from build123d import *

# Parameters (mm, degrees)
SKETCH2_W           = 219.964
SKETCH2_H           = 149.86
SKETCH1_W           = 190.5
SKETCH1_H           = 116.84
SKETCH2_2_W         = 219.964
SKETCH2_2_H         = 149.86
BOSS_EXTRUDE2_DEPTH = 4.572
SKETCH3_W           = 177.8
SKETCH3_H           = 109.22
BOSS_EXTRUDE3_DEPTH = 5.08
SKETCH4_W           = 167.64
SKETCH4_H           = 99.06
CUT_EXTRUDE1_DEPTH  = 6.08
SKETCH4_2_W         = 167.64
SKETCH4_2_H         = 99.06
CUT_EXTRUDE2_DEPTH  = 8.89
SKETCH5_R           = 6.35
CUT_EXTRUDE3_DEPTH  = 19.05


with BuildPart() as part:
    # Sketch2 → Loft1 section 0
    with BuildSketch(Plane(origin=(0, 12.0904, 0), x_dir=(1, 0, 0), z_dir=(0, 1, 0))):
        with Locations((-109.982, -58.640869565)):
            Rectangle(SKETCH2_W, SKETCH2_H)
    # Sketch1 → Loft1 section 1
    with BuildSketch(Plane(origin=(0, 0, 0), x_dir=(1, 0, 0), z_dir=(0, 1, 0))):
        with Locations((-95.25, -58.42)):
            Rectangle(SKETCH1_W, SKETCH1_H)
    loft()

    # Sketch2_2 → Boss-Extrude2 (add)
    with BuildSketch(Plane(origin=(0, 12.0904, 0), x_dir=(1, 0, 0), z_dir=(0, 1, 0))):
        with Locations((-109.982, -58.640869565)):
            Rectangle(SKETCH2_2_W, SKETCH2_2_H)
    extrude(amount=BOSS_EXTRUDE2_DEPTH)

    # Sketch3 → Boss-Extrude3 (add)
    with BuildSketch(Plane(origin=(0, 16.51, 0), x_dir=(1, 0, 0), z_dir=(0, 1, 0))):
        with Locations((-97.79, -58.640869565)):
            Rectangle(SKETCH3_W, SKETCH3_H)
    extrude(amount=BOSS_EXTRUDE3_DEPTH)

    # Sketch4 → Cut-Extrude1 (cut, through all)
    with BuildSketch(Plane(origin=(0, 16.51, 0), x_dir=(1, 0, 0), z_dir=(0, 1, 0))):
        with Locations((-97.79, -58.640869565)):
            Rectangle(SKETCH4_W, SKETCH4_H)
    extrude(amount=CUT_EXTRUDE1_DEPTH, mode=Mode.SUBTRACT)

    # Sketch4_2 → Cut-Extrude2 (cut)
    with BuildSketch(Plane(origin=(0, 16.51, 0), x_dir=(1, 0, 0), z_dir=(0, 1, 0))):
        with Locations((-97.79, -58.640869565)):
            Rectangle(SKETCH4_2_W, SKETCH4_2_H)
    extrude(amount=-CUT_EXTRUDE2_DEPTH, mode=Mode.SUBTRACT)

    # Sketch5 → Cut-Extrude3 (cut)
    with BuildSketch(Plane(origin=(0, 0, 0), x_dir=(0, 0, -1), z_dir=(1, 0, 0))):
        with Locations((-82.770869565, 16.6624)):
            Circle(SKETCH5_R)
        with Locations((-34.510869565, 16.51)):
            Circle(SKETCH5_R)
    extrude(amount=-CUT_EXTRUDE3_DEPTH, mode=Mode.SUBTRACT)


solid = part.part
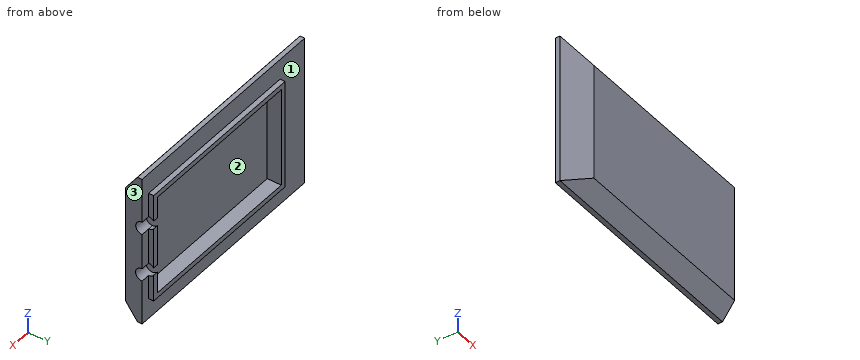
Design review of the part built by this model. Coordinates are the model's own, in mm. Face numbers are marked on the shaded views. Round coordinates to 2 decimals unless told otherwise and drop trailing zeros. Answer as a JSON object with one key per item and string values.
Item 1: Wall thickness on L1, parallel to Z at x = -7.5, y = 16.51; L2, parallel to Z at x = -153, y = 18.5; L3, parallel to Z at x = -88.5, y = 14: over which ranges is each line inside the solid? List them lowest first. Write a range as from..to.
Answer sheet:
{"L1": "z = -16.29..28.16, 40.86..76.42, 89.12..133.57", "L2": "z = 4.03..9.11, 108.17..113.25", "L3": "z = -16.29..9.11, 108.17..133.57"}
Item 2: The part is to be moulded in two halves that separate along X. For the marked faces 1, 2 and 3, say which applies: pulls with the +X half, pulls with the -X half, needs draft (parallel to the pull), parting line crosses it, or undercut.
Answer sheet:
{"face 1": "needs draft", "face 2": "undercut", "face 3": "pulls with the +X half"}
Item 3: Clearance check with flat-ended pins moving along their axes: P1, Ø3, axis at x = -107, y = 8, coming from the -Z side; P2, Ø1.5, axis at x = -65.5, y = 18, coming from the +Z side; P3, Ø2.5, axis at y = 18, z = 60, coming from the -X side. State where each tip first meets the part, or that it passes through.
Answer sheet:
{"P1": "stops at z = -12.8", "P2": "stops at z = 113.25", "P3": "stops at x = -186.69"}
